```python
from build123d import *

# Parameters (mm, degrees)
SKETCH_1_R               = 9
EXTRUDE_1_DEPTH          = 52
SKETCH_2_R               = 7.8
EXTRUDE_2_DEPTH          = 12
EXTRUDE_3_DEPTH          = 1.8
EXTRUDE_3_DEPTH_BACK     = 1.8
SKETCH_3_R               = 2.6
EXTRUDE_4_DEPTH          = 1.8
EXTRUDE_4_DEPTH_BACK     = 1.8
SKETCH_4_R               = 1.6
CUT_EXTRUDE_1_DEPTH      = 26
CUT_EXTRUDE_1_DEPTH_BACK = 75
SKETCH_5_R               = 12.444758302
SKETCH_5_R_2             = 7.5
CUT_EXTRUDE_2_DEPTH      = 75
CUT_EXTRUDE_2_DEPTH_BACK = 15
SKETCH_6_R               = 11.570191829


with BuildPart() as part:
    # Sketch 1 → Extrude 1 (new body)
    with BuildSketch(Plane(origin=(0, 0, 0), x_dir=(1, 0, 0), z_dir=(0, 1, 0))):
        with Locations(Location((0, 0, 0), (0, 0, 90))):
            Circle(SKETCH_1_R)
    extrude(amount=EXTRUDE_1_DEPTH)

    # Sketch 2 → Extrude 2 (add)
    with BuildSketch(Plane(origin=(0, 52, 0), x_dir=(1, 0, 0), z_dir=(0, 1, 0))):
        with Locations(Location((0, 0, 0), (0, 0, 270))):
            Circle(SKETCH_2_R)
    extrude(amount=EXTRUDE_2_DEPTH)

    # Sketch 3 → Extrude 3 (add, two sides: drawn at the far end of the back side and taken through both)
    with BuildSketch(Plane.XY.offset(-EXTRUDE_3_DEPTH_BACK)):
        with BuildLine():
            Line((-4.255, 59.5), (4.255, 59.5))
            Line((4.255, 59.5), (4.255, 68.5))
            ThreePointArc((4.255, 68.5), (0, 72.755), (-4.255, 68.5))
            Line((-4.255, 68.5), (-4.255, 59.5))
        make_face()
        with Locations((0, 68.5)):
            Circle(SKETCH_3_R, mode=Mode.SUBTRACT)
    extrude(amount=EXTRUDE_3_DEPTH + EXTRUDE_3_DEPTH_BACK)

    # Sketch 4 → Extrude 4 (add, two sides: drawn at the far end of the back side and taken through both)
    with BuildSketch(Plane.XY.offset(-EXTRUDE_4_DEPTH_BACK)):
        with BuildLine():
            Line((-4.65, -16.5), (-4.65, -8.5))
            Line((-4.65, -8.5), (-4.65, 0))
            Line((-4.65, 0), (4.65, 0))
            Line((4.65, 0), (4.65, -8.5))
            Line((4.65, -8.5), (4.65, -16.5))
            ThreePointArc((4.65, -16.5), (0, -21.15), (-4.65, -16.5))
        make_face()
        with Locations((0, -16.5)):
            Circle(SKETCH_4_R, mode=Mode.SUBTRACT)
    extrude(amount=EXTRUDE_4_DEPTH + EXTRUDE_4_DEPTH_BACK)

    # Sketch 5 → Cut-Extrude 1 (cut, two sides: drawn at the far end of the back side and taken through both)
    with BuildSketch(Plane.XZ.offset(-CUT_EXTRUDE_1_DEPTH_BACK)):
        Circle(SKETCH_5_R)
        with Locations(Location((0, 0, 0), (0, 0, 90))):
            Circle(SKETCH_5_R_2, mode=Mode.SUBTRACT)
    extrude(amount=CUT_EXTRUDE_1_DEPTH + CUT_EXTRUDE_1_DEPTH_BACK, mode=Mode.SUBTRACT)

    # Sketch 6 → Cut-Extrude 2 (cut, two sides: drawn at the far end of the back side and taken through both)
    with BuildSketch(Plane(origin=(0, 64, 0), x_dir=(1, 0, 0), z_dir=(0, 1, 0)).offset(-CUT_EXTRUDE_2_DEPTH_BACK)):
        Circle(SKETCH_6_R)
    extrude(amount=CUT_EXTRUDE_2_DEPTH + CUT_EXTRUDE_2_DEPTH_BACK, mode=Mode.SUBTRACT)


solid = part.part
```
CAD build for the part. Positions are in the model's coordinates, mm. A direction names the side the tool comes from. Coordinates: 2 decimals unless noted, no trailing zeros. Order: outer loops, then holes, each group sorted by start corner. A loop starts at its lowest first (then second) coordinate and runs counter-clockwise, first axis right, second up.
(1) Saw through at B-B, the plane z = 0. Write the cut outline in (x, y).
Solution:
outline: (-7.5, 0) - (-4.65, 0) - (-4.65, -16.5) arc R4.65 ccw to (4.65, -16.5) - (4.65, 0) - (7.5, 0) - (7.5, 49) - (-7.5, 49) - close; hole circle Ø3.2 at (0, -16.5)
(2) Saw through at A-A, the plane x = 0. Write the cut outline in (y, z).
Solution:
outline: (-21.15, -1.8) - (-18.1, -1.8) - (-18.1, 1.8) - (-21.15, 1.8) - close; (-14.9, -1.8) - (0, -1.8) - (0, -7.5) - (49, -7.5) - (49, 7.5) - (0, 7.5) - (0, 1.8) - (-14.9, 1.8) - close
(3) Mould opens along X. For faces 1 (the face through (0.1, -21.15, -0.03)), 2 (the face through (0, -10, -1.8)), 3 (the face through (-0.208, -14.914, -0.025)) say: released by +X, released by -X, zero draft, split by the parting line, or undercut.
Solution:
face 1: split by the parting line
face 2: zero draft
face 3: undercut
(4) Drill centre lines: L1, parallel to Y at x = 0, z = 0.6; L2, parallel to Y at x = -1.5, z = -5; L3, parallel to Z at x = -0.75, y = -8.5. Where is each one in solid material? Low to high.
Solution:
L1: y = -21.15 to -18.1, -14.9 to 49
L2: y = 0 to 49
L3: z = -1.8 to 1.8
(5) Saw through at D-D, the plane x = -3.25. Write the cut outline in (y, z), and give its area (3 significant figures).
Solution:
outline: (-19.83, -1.8) - (0, -1.8) - (0, -6.76) - (49, -6.76) - (49, 6.76) - (0, 6.76) - (0, 1.8) - (-19.83, 1.8) - close
area: 734 mm2
(6) Pin check, flat tips, straight feed: pin 1 Ø1.1 at (y, z) = (-7.5, -0.5) entering from -X; pin 2 Ø6 at (x, y) = (-4.5, -10.5) entering from -Z; pin 3 Ø8 at (y, z) = (-10.5, -3) entering from +X; pin 4 Ø5 at (y, z) = (31.5, 1.5) entering from -X. Stop position of each tip, or through.
Solution:
pin 1: stops at x = -4.65
pin 2: stops at z = -1.8
pin 3: stops at x = 4.65
pin 4: stops at x = -7.5
(7) Saw through at C-C, the plane y = 22.5. Write the cut outline in (x, z), and give its area (3 significant figures).
Solution:
outline: circle Ø15 at (0, 0)
area: 177 mm2
(8) Which spindle directions (+Z, -Z, +X, -X, +Y, -Y) get a long thin tool onto all of the face, cutting with end or side? Do faces 4 (the face through (0, -10, 1.8)), 5 (the face through (4.65, -8, 0)), 6 (the face through (-4.65, -8, 0)). Say none if no direction does.
Solution:
face 4: +Z, +X, -X, -Y
face 5: +Z, -Z, +X, -Y
face 6: +Z, -Z, -X, -Y
